Check sheet for the modelled part. Datum: model origin and axes. Units: mm. A direction names the side the tool comes from. Coordinates: 2 decimals unless noted, no trailing zeros. Loops run counter-clockwise (first coordinate to the right, second up) from the corner with the lowest first, then second, coordinate; pieces in that order, holes last. Notation, with made-up numbers: (19.5, 66.25) -> (68.5, 66.25) arc R35 cw to (68.5, 98.25) -> close; hole circle Ø2 at (62, 64). An arc over 180 degrees is marked (long way). Use CSV: the item, a comma, the result in double quotes.
Autodesk Inventor part; units mm, degrees
ref_plane "YZ Plane" through (0, 0, 0) normal (1, 0, 0) x (0, 1, 0)
ref_plane "XZ Plane" through (0, 0, 0) normal (0, 1, 0) x (-1, 0, 0)
ref_plane "XY Plane" through (0, 0, 0) normal (0, 0, 1) x (1, 0, 0)
sketch "Base" plane through (0, 0, 0) normal (0, 1, 0) x (-1, 0, 0)
  line L0 (-40, 50) -> (40, 50)
  line L1 (40, 50) -> (40, -50)
  line L2 (40, -50) -> (-40, -50)
  line L3 (-40, -50) -> (-40, 50)
  line L4 (-40, 50) -> (40, -50) construction
  line L5 (40, 50) -> (-40, -50) construction
  circle A0 centre (10, 40) radius 5
  circle A1 centre (-10, 40) radius 5
  circle A2 centre (10, -40) radius 5
  circle A3 centre (-10, -40) radius 5
  circle A4 centre (-30, 30) radius 1.275
  circle A5 centre (-30, -30) radius 1.275
  circle A6 centre (30, 0) radius 1.275
  line L6 (38, -48) -> (38, 48)
  line L7 (38, 48) -> (-38, 48)
  line L8 (-38, 48) -> (-38, -48)
  line L9 (-38, -48) -> (38, -48)
  point P0 (0, 0)
  dimension "d0" = 80
  dimension "d1" = 100
  dimension "d2" = 30
  dimension "d3" = 10
  dimension "d4" = 10
  dimension "d6" = 10
  dimension "d7" = 2.55
  dimension "d8" = 70
  dimension "d10" = 2.55
  dimension "d11" = 2
extrude "Extrusión base" add sketch "Base" along normal blind 2 contours L9 L8 L7 L6
extrude "Paredes" add sketch "Base" along normal blind 40 contours L0 L1 L2 L3
sketch "Boceto2" plane through (-40, 0, -50) normal (-1, 0, 0) x (0, 0, 1)
  line L0 (0, 40) -> (100, 40)
  line L1 (98, 40) -> (2, 40)
  line L2 (46.25, 35) -> (53.75, 35)
  line L3 (53.75, 35) -> (53.75, 40)
  line L4 (53.75, 40) -> (46.25, 40)
  line L5 (46.25, 40) -> (46.25, 35)
  line L6 (46.25, 35) -> (53.75, 40) construction
  line L7 (53.75, 35) -> (46.25, 40) construction
  point P0 (50, 0)
  point P1 (50, 37.5)
  dimension "d16" = 2.5
  dimension "d17" = 7.5
extrude "Extrusión3" add sketch "Boceto2" along normal blind 2
mirror "Simetría1" about plane through (0, 0, 0) normal (1, 0, 0) of "Extrusión3"
sketch "Boceto3" plane through (-42, 0, -50) normal (-1, 0, 0) x (0, 0, 1)
  line L0 (53.75, 40) -> (46.25, 40)
  line L1 (53.75, 40) -> (53.75, 35)
  line L2 (46.25, 38) -> (53.75, 38)
  line L3 (53.75, 38) -> (53.75, 40)
  line L4 (53.75, 40) -> (46.25, 40)
  line L5 (46.25, 40) -> (46.25, 38)
  line L6 (46.25, 38) -> (53.75, 40) construction
  line L7 (53.75, 38) -> (46.25, 40) construction
  point P0 (50, 0)
  point P1 (50, 39)
  dimension "d20" = 1
extrude "Extrusión4" add sketch "Boceto3" along normal blind 8
mirror "Simetría2" about plane through (0, 0, 0) normal (1, 0, 0) of "Extrusión4"
sketch "Boceto4" plane through (0, 40, 0) normal (0, 1, 0) x (1, 0, 0)
  line L0 (-50, -3.75) -> (-50, 3.75)
  line L1 (-40, -3.75) -> (-50, -3.75)
  circle A0 centre (-45, 0) radius 1.275
  point P0 (0, 0)
  dimension "d23" = 5
  dimension "d24" = 3.75
  dimension "d25" = 2.55
hole "Agujero1" at (-45, 40, 0) direction (0, -1, 0) diameter 2.55 end through all
mirror "Simetría3" about plane through (0, 0, 0) normal (1, 0, 0) of "Agujero1"
properties part number "Contenedor Puente H v1.0"
1) Cross-section at C-C on x = 30. Record the boundary of the cut face in (y, z) (3 decimals).
Answer below:
outline,"(0, -50) -> (40, -50) -> (40, -48) -> (2, -48) -> (2, -31.275) -> (0, -31.275) -> close; (0, -28.725) -> (2, -28.725) -> (2, 28.725) -> (0, 28.725) -> close; (0, 31.275) -> (2, 31.275) -> (2, 48) -> (40, 48) -> (40, 50) -> (0, 50) -> close"
2) Go/stop test with flat-tipped pins: pin 1 Ø2 at (x, z) = (-2.5, 35) entering from +Y; pin 2 Ø5.5 at (x, y) = (44.5, 37) entering from -Z; pin 3 Ø19 at (y, z) = (16.5, -2) entering from +X; pin 4 Ø2 at (x, z) = (30, -30) entering from +Y. Record where each tip stops, or that it passes through.
Answer below:
pin 1,"stops at y = 2"
pin 2,"stops at z = -3.75"
pin 3,"stops at x = 40"
pin 4,"passes through"
3) Cross-section at D-D on z = 30. Record the boundary of the cut face in (x, y) (3 decimals).
Answer below:
outline,"(-40, 0) -> (28.725, 0) -> (28.725, 2) -> (-38, 2) -> (-38, 40) -> (-40, 40) -> close; (31.275, 0) -> (40, 0) -> (40, 40) -> (38, 40) -> (38, 2) -> (31.275, 2) -> close"
4) Cross-section at A-A on y = 27. Record the boundary of the cut face in (x, z).
Answer below:
outline,"(-40, -50) -> (40, -50) -> (40, 50) -> (-40, 50) -> close; hole (-38, -48) -> (38, -48) -> (38, 48) -> (-38, 48) -> close"
5) Access from +Z, -Z, +X, -X, +Y, -Y to the whole of each face (thin tool, end or side, straight path). Record for faces 3 (the flat face through (47, 38, 0)), 4 (the flat face through (38, 21, 1)), 5 (the flat face through (44, 39, 3.75)), 6 (the flat face through (-47, 38, 0)).
Answer below:
face 3,"+Z, -Z, +X, -Y"
face 4,"+Y"
face 5,"+Z, +X, +Y, -Y"
face 6,"+Z, -Z, -X, -Y"
6) Cross-section at B-B on x = 45. Record the boundary of the cut face in (y, z) (3 decimals), and give its area (3 significant figures).
Answer below:
outline,"(38, -3.75) -> (40, -3.75) -> (40, -1.275) -> (38, -1.275) -> close; (38, 1.275) -> (40, 1.275) -> (40, 3.75) -> (38, 3.75) -> close"
area,"9.90 mm²"
7) Draft check along X on faces 1 (the cylindrical face through (-13, 1, -44)), 2 (the flat face through (-44, 39, 3.75)). Enter one of: released by +X, released by -X, zero draft, split by the parting line, or undercut.
Answer below:
face 1,"undercut"
face 2,"zero draft"
8) Thickness scan on line 1 along X through (y, z) = (39, 0) (3 decimals); line 2 along Z through (x, y) = (30, 1.3) (3 decimals); line 3 along Z through (x, y) = (-33.5, 36). Record the ranges inside material, lowest first. Write a range as from..to.
Answer below:
line 1,"x = -50..-46.275, -43.725..-38, 38..43.725, 46.275..50"
line 2,"z = -50..-31.275, -28.725..28.725, 31.275..50"
line 3,"z = -50..-48, 48..50"
